from build123d import *

# Parameters (mm, degrees)
SKETCH1_R               = 24
BOSS_EXTRUDE1_DEPTH     = 5
EXTRUDE_THIN1_DEPTH     = 5
SKETCH4_W               = 33
SKETCH4_H               = 10
BOSS_EXTRUDE2_DEPTH     = 5
SKETCH5_R               = 22
SKETCH5_W               = 33
SKETCH5_H               = 5
CUT_EXTRUDE1_DEPTH      = 26.5
SKETCH6_R               = 1.6
CUT_EXTRUDE2_DEPTH      = 20
CUT_EXTRUDE2_DEPTH_BACK = 10
SKETCH7_R               = 2.4
CUT_EXTRUDE3_DEPTH      = 5
FILLET3_R               = 5


with BuildPart() as part:
    # Sketch1 → Boss-Extrude1 (new body, symmetric)
    with BuildSketch(Plane.XY):
        Circle(SKETCH1_R)
    extrude(amount=BOSS_EXTRUDE1_DEPTH, both=True)

    # Sketch2 → Extrude-Thin1 (add, symmetric)
    with BuildSketch(Plane.XY):
        with BuildLine():
            Line((-39.748737342, -26.748737342), (-25.162950904, -26.748737342))
            ThreePointArc((-25.162950904, -26.748737342), (-24.014900607, -26.520375939), (-23.04163056, -25.870057685))
            Line((-23.04163056, -25.870057685), (0, -2.828427125))
            Line((0, -2.828427125), (23.04163056, -25.870057685))
            ThreePointArc((23.04163056, -25.870057685), (24.014900607, -26.520375939), (25.162950904, -26.748737342))
            Line((25.162950904, -26.748737342), (39.748737342, -26.748737342))
            Line((39.748737342, -26.748737342), (39.748737342, -22.748737342))
            Line((39.748737342, -22.748737342), (25.577164466, -22.748737342))
            Line((25.577164466, -22.748737342), (0, 2.828427125))
            Line((0, 2.828427125), (-25.577164466, -22.748737342))
            Line((-25.577164466, -22.748737342), (-39.748737342, -22.748737342))
            Line((-39.748737342, -22.748737342), (-39.748737342, -26.748737342))
        make_face()
    extrude(amount=EXTRUDE_THIN1_DEPTH, both=True)

    # Sketch4 → Boss-Extrude2 (add, symmetric)
    with BuildSketch(Plane.XY):
        with Locations((-16.5, 0)):
            Rectangle(SKETCH4_W, SKETCH4_H)
    extrude(amount=BOSS_EXTRUDE2_DEPTH, both=True)

    # Sketch5 → Cut-Extrude1 (cut)
    with BuildSketch(Plane.XY.offset(5)):
        Circle(SKETCH5_R)
        with Locations((-16.5, 0)):
            Rectangle(SKETCH5_W, SKETCH5_H)
    extrude(amount=-CUT_EXTRUDE1_DEPTH, mode=Mode.SUBTRACT)

    # Sketch6 → Cut-Extrude2 (cut, two sides)
    with BuildSketch(Plane(origin=(0, 5, 0), x_dir=(1, 0, 0), z_dir=(0, 1, 0))) as cut_extrude2_sk:
        with Locations((-29, 0)):
            Circle(SKETCH6_R)
    extrude(amount=CUT_EXTRUDE2_DEPTH, mode=Mode.SUBTRACT)
    extrude(cut_extrude2_sk.sketch, amount=-CUT_EXTRUDE2_DEPTH_BACK, mode=Mode.SUBTRACT)

    # Sketch7 → Cut-Extrude3 (cut, through all)
    with BuildSketch(Plane(origin=(0, -22.748737342, 0), x_dir=(1, 0, 0), z_dir=(0, 1, 0))):
        with Locations((-32.748737342, 0)):
            Circle(SKETCH7_R)
        with Locations((32.748737342, 0)):
            Circle(SKETCH7_R)
    extrude(amount=-CUT_EXTRUDE3_DEPTH, mode=Mode.SUBTRACT)

    # Fillet3
    fillet3_edges = [part.edges().sort_by_distance(p)[0] for p in [
        (-15.497320963, -18.325748088, 0),
        (15.497320963, -18.325748088, 0),
        (18.325748088, -15.497320963, 0),
        (-18.325748088, -15.497320963, 0),
    ]]
    fillet(fillet3_edges, radius=FILLET3_R)


solid = part.part
Check sheet for the modelled part. Datum: model origin and axes. Units: mm. A direction names the side the tool comes from. Give positions to 0.01 mm unless a question says otherwise; leave off trailing zeros. Write each loop counter-clockwise with the first axis right and the second up, starting at its lowest first coordinate (ties: lowest second). Pieces come first, ordered by that corner, then holes. Notation, with made-up numbers: (-40, -12.5) -> (-18, -12.5) arc R21 ccw to (-18, -4.5) -> close; hole circle Ø10 at (-5.75, 88). An arc over 180 degrees is marked (long way). One line per item, written item: value. Start each with the question number.
Item 1: Material ranges on probe 1 along Y at (x, z) = (-26.5, 4); probe 2 along Z at (x, y) = (-29, 4.1); probe 3 along X at (y, z) = (-25.4, 0), recorded low to high. Write a range as from..to.
Item 2: Section check C-C on y = 17. Record the cut outline in (x, z), then the cut area to 3 significant figures.
Item 3: Section check B-B on x = -29. Record the cut outline in (y, z).
Item 4: Draft check along Z on faces 1 (the flat face through (-27, 5, 0)), 2 (the cylindrical face through (30.35, -24.72, -0.11)). Enter one of: +Z half, -Z half, draft (parallel to the pull), parting line (faces both ways), or undercut.
Item 5: Section check A-A on x = 0. Record the cut outline in (y, z).
Item 6: Gauge pin test, flat ends, axial feed: pin 1 (5.5 mm diameter, centred on x = -32.75, z = 0, fed in from +Y); pin 2 (1 mm diameter, centred on y = -1.5, z = 1.5, fed in from -X); pin 3 (1.5 mm diameter, centred on x = -18.5, z = 0, fed in from -Y). Record the tip position at first contact, or that the pin passes through.
Item 7: Section check D-D on z = -4. Record the cut outline in (x, y).
Item 8: Tool access check on faces 3 (the flat face through (-33, -4, 0)), 4 (the cylindrical face through (21.98, -0.93, 0.07)), 5 (the flat face through (-27, -5, 0)), 6 (the cylindrical face through (-24.03, -26.527, 0.07)), 7 (the flat face through (39.749, -25, 0)). Record the directions out of +Z, -Z, +X, -X, +Y, -Y that give a thin tool (end or side, any length) a straight path to the whole face; none if there is none.
Results list:
1. probe 1: -26.75..-22.75, -5..-2.5, 2.5..5
1. probe 2: -5..-1.6, 1.6..5
1. probe 3: -39.75..-35.15, -30.35..-22.57, 22.57..30.35, 35.15..39.75
2. outline: (-16.94, -5) -> (-13.96, -5) -> (-13.96, 5) -> (-16.94, 5) -> close; (13.96, -5) -> (16.94, -5) -> (16.94, 5) -> (13.96, 5) -> close
2. area: 59.5 mm²
3. outline: (-26.75, -5) -> (-22.75, -5) -> (-22.75, 5) -> (-26.75, 5) -> close; (-5, -5) -> (-2.5, -5) -> (-2.5, -1.6) -> (-5, -1.6) -> close; (-5, 1.6) -> (-2.5, 1.6) -> (-2.5, 5) -> (-5, 5) -> close; (2.5, -5) -> (5, -5) -> (5, -1.6) -> (2.5, -1.6) -> close; (2.5, 1.6) -> (5, 1.6) -> (5, 5) -> (2.5, 5) -> close
4. face 1: draft
4. face 2: undercut
5. outline: (-24, -5) -> (-22, -5) -> (-22, 5) -> (-24, 5) -> close; (22, -5) -> (24, -5) -> (24, 5) -> (22, 5) -> close
6. pin 1: y = 5
6. pin 2: x = 21.91
6. pin 3: y = -22.08
7. outline: (-39.75, -26.75) -> (-25.16, -26.75) arc R3 ccw to (-23.04, -25.87) -> (-18.49, -21.31) arc R5 cw to (-12.37, -20.57) arc R24 ccw to (12.37, -20.57) arc R5 cw to (18.49, -21.31) -> (23.04, -25.87) arc R3 ccw to (25.16, -26.75) -> (39.75, -26.75) -> (39.75, -22.75) -> (25.58, -22.75) -> (21.31, -18.49) arc R5 cw to (20.57, -12.37) arc R24 ccw (long way) to (-23.47, 5) -> (-33, 5) -> (-33, 2.5) -> (-21.86, 2.5) arc R22 cw (long way) to (-21.86, -2.5) -> (-33, -2.5) -> (-33, -5) -> (-23.47, -5) arc R24 ccw to (-20.57, -12.37) arc R5 cw to (-21.31, -18.49) -> (-25.58, -22.75) -> (-39.75, -22.75) -> close
8. face 3: +Z, -Z, -X, +Y
8. face 4: +Z, -Z
8. face 5: +Z, -Z, -X
8. face 6: +Z, -Z, -Y
8. face 7: +Z, -Z, +X, +Y, -Y
